Check sheet for the modelled part. Datum: model origin and axes. Units: mm. Face numbers are marked on the shaded views. A direction names the side the tool comes from. Give positions to 0.01 mm unless a question says otherwise; leave off trailing zeros. Write each loop counter-clockwise with the first axis right and the second up, starting at its lowest first coordinate (ties: lowest second). Pieces come first, ordered by that corner, then holes. Notation, with made-up numbers: M 50.5,-39.5 L 108.5,-39.5 A15 cw 108.5,-19.5 Z; hole C 53,33.5 d10. An arc over 180 degrees is marked long. One line per item, written item: value. Start each with the question number.
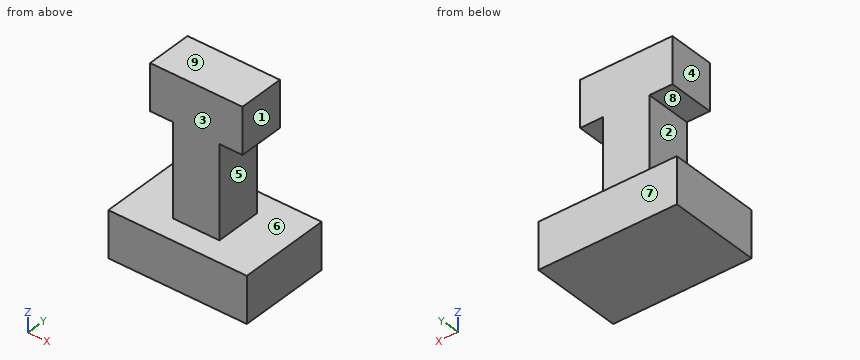
from build123d import *

# Parameters (mm, degrees)
F1_DEPTH = 20
F2_DEPTH = 10


with BuildPart() as f1:
    # F0 (on Front) → F1 (new body, symmetric)
    with BuildSketch(Plane.XZ):
        Polygon((0, 20), (0, 0), (60, 0), (60, 20), (40, 20), (20, 20), align=None)
    extrude(amount=F1_DEPTH, both=True)

    # F0 (on Front) → F2 (join, symmetric)
    with BuildSketch(Plane.XZ):
        Polygon((20, 60), (20, 20), (40, 20), (40, 60), (50, 60), (50, 80), (10, 80), (10, 60), align=None)
    extrude(amount=F2_DEPTH, both=True)


solid = f1.part
1) Cross-section at D-D (z = 33). Record the boundary of the cut face in (x, y).
2) Gauge pin test, flat ends, axial feed: pin 1 (3 mm diameter, centred on x = 16, y = -0.5, fed in from -Z); pin 2 (6 mm diameter, centred on y = 1.5, z = 70.5, fed in from -X); pin 3 (4 mm diameter, centred on y = -9.5, z = 65, fed in from +X); pin 4 (1.5 mm diameter, centred on x = 51.5, y = 2, fed in from +Z). Record the tip position at first contact, or that the pin passes through.
3) Cross-section at B-B (y = -1.5). Record the boundary of the cut face in (x, z).
4) Material ranges on L1, parallel to Z at x = 49.5, y = -2.5; L2, parallel to Y at x = 17.5, z = 76; L3, parallel to Z at x = 3, y = 2, recorded low to high. Write a range as from..to.
5) Tool access check on the marked faces 1, 2, 3, 4 and 5. Record the directions out of +Z, -Z, +X, -X, +Y, -Y that give a thin tool (end or side, any length) a straight path to the whole face; none if there is none.
6) Cross-section at A-A (x = 43). Record the boundary of the cut face in (y, z), plus the area to 3 significant figures.
7) Draft check along Z on the marked faces 6, 7, 8 and 9. Enter one of: released by +Z, released by -Z, zero draft, split by the parting line, or undercut.
8) Cross-section at C-C (x = 30). Record the boundary of the cut face in (y, z).
Data:
1. outline: M 20,-10 L 40,-10 L 40,10 L 20,10 Z
2. pin 1: stops at z = 0
2. pin 2: stops at x = 10
2. pin 3: stops at x = 50
2. pin 4: stops at z = 20
3. outline: M 0,0 L 60,0 L 60,20 L 40,20 L 40,60 L 50,60 L 50,80 L 10,80 L 10,60 L 20,60 L 20,20 L 0,20 Z
4. L1: z = 0..20, 60..80
4. L2: y = -10..10
4. L3: z = 0..20
5. face 1: +Z, +X, +Y, -Y
5. face 2: -X, +Y, -Y
5. face 3: +Z, +X, -X, -Y
5. face 4: +Z, -X, +Y, -Y
5. face 5: +X, +Y, -Y
6. outline: M -20,0 L 20,0 L 20,20 L -20,20 Z; M -10,60 L 10,60 L 10,80 L -10,80 Z
6. area: 1,200 mm2
7. face 6: undercut
7. face 7: zero draft
7. face 8: undercut
7. face 9: released by +Z
8. outline: M -20,0 L 20,0 L 20,20 L 10,20 L 10,80 L -10,80 L -10,20 L -20,20 Z
